Build history of the part. All positions in model axes, mm. Face numbers are marked on the shaded views. A direction names the side the tool comes from. Round coordinates to 2 decimals unless told otherwise and drop trailing zeros. Order: outer loops, then holes, each group sorted by start corner. A loop starts at its lowest first (then second) coordinate and runs counter-clockwise, first axis right, second up. Notation, with made-up numbers: (0, 56) -> (11, 56) arc R11 cw to (11, 69) -> close; hole circle Ø8 at (-36, 67). An arc over 180 degrees is marked (long way). Use a Markdown table: item, result. Add a question column.
Item 1: Probe L1, parallel to Y at x = 0, z = -2; L2, parallel to X at y = 7.5, z = 0.5; L3, parallel to Z at x = 15.5, y = 21.5. List the from-to ranges inside material, lowest first.
Item 2: Pin check, flat tips, straight feed: pin 1 (3 mm diameter, centred on x = -11, z = -2, fed in from +Y); pin 2 (2 mm diameter, centred on x = 9, z = 0.5, fed in from -Y); pin 3 (1 mm diameter, centred on x = 18, z = -0.5, fed in from -Y). Stop position of each tip, or through.
Item 3: Slice it at B-B, the plane x = 0. Give the cut face in (y, z), plus the area to 3 significant figures.
Item 4: Two-plate mould, pull along Y, no slides. Class the marked faces 1, 2 and 3: released by +Y, released by -Y, zero draft, split by the parting line, or undercut.
Item 5: Slice it at C-C, the plane y = 7. Give the cut face in (x, z).
Item 6: Slice it at A-A, the plane y = 0. Give the cut face in (x, z), plus the area to 3 significant figures.
Item 7: Slice it at D-D, the plane z = 2.25. Give the cut face in (x, y).
Item 8: 3-axis set-ups, long thin cutter, end or side, ignore diameter. For the marked faces 4 and 5: which of +Z, -Z, +X, -X, +Y, -Y reach the whole face in a straight line?
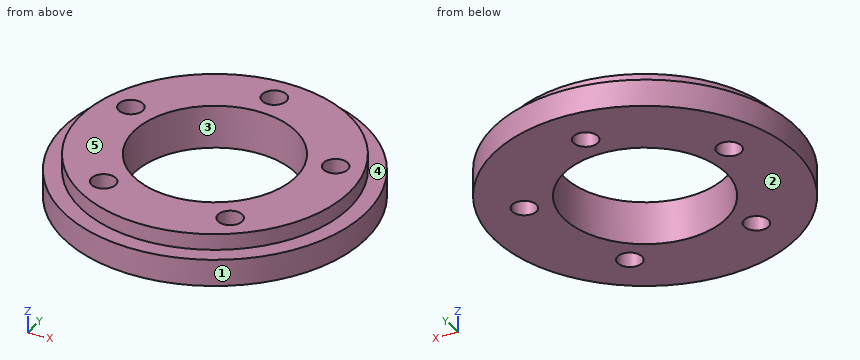
Autodesk Inventor part; units mm, degrees
ref_plane "YZ Plane" through (0, 0, 0) normal (1, 0, 0) x (0, 1, 0)
ref_plane "XZ Plane" through (0, 0, 0) normal (0, 1, 0) x (-1, 0, 0)
ref_plane "XY Plane" through (0, 0, 0) normal (0, 0, 1) x (1, 0, 0)
sketch "스케치1" plane through (0, 0, 0) normal (0, 0, 1) x (1, 0, 0)
  circle A0 centre (0, 0) radius 24.9
  circle A1 centre (0, 0) radius 28
  circle A2 centre (0, 0) radius 15
  dimension "d0" = 49.8
  dimension "d1" = 56
  dimension "d2" = 30
extrude "돌출1" add sketch "스케치1" along normal blind 3 contours A0
extrude "돌출2" add sketch "스케치1" against normal blind 5 contours A0 | A1
sketch "스케치3" plane through (0, 0, 3) normal (0, 0, 1) x (1, 0, 0)
  circle A0 centre (0, 0) radius 20 construction
  circle A1 centre (0, 20) radius 2.25
  circle A2 centre (-19.0211, 6.1803) radius 2.25
  circle A3 centre (-11.7557, -16.1803) radius 2.25
  circle A4 centre (11.7557, -16.1803) radius 2.25
  circle A5 centre (19.0211, 6.1803) radius 2.25
  dimension "d9" = 40
  dimension "d10" = 4.5
  dimension "d13" = 360
extrude "돌출3" cut sketch "스케치3" against normal blind 44.5
properties part number "사이클로이드 기어 축 연결 하우징"
Check sheet entries:
| question | item | result |
|---|---|---|
| 1 | L1 | -28 to -15, 15 to 17.75, 22.25 to 28 |
| 1 | L2 | -23.74 to -20.84, -17.2 to -12.99, 12.99 to 17.2, 20.84 to 23.74 |
| 1 | L3 | -5 to 0 |
| 2 | pin 1 | y = 26.34 |
| 2 | pin 2 | y = -26.79 |
| 2 | pin 3 | y = -21.86 |
| 3 | outline | (-28, -5) -> (-15, -5) -> (-15, 3) -> (-24.9, 3) -> (-24.9, 0) -> (-28, 0) -> close; (15, -5) -> (17.75, -5) -> (17.75, 3) -> (15, 3) -> close; (22.25, -5) -> (28, -5) -> (28, 0) -> (24.9, 0) -> (24.9, 3) -> (22.25, 3) -> close |
| 3 | area | 153 mm2 |
| 4 | face 1 | split by the parting line |
| 4 | face 2 | zero draft |
| 4 | face 3 | undercut |
| 5 | outline | (-27.11, -5) -> (-21.12, -5) -> (-21.12, 3) -> (-23.9, 3) -> (-23.9, 0) -> (-27.11, 0) -> close; (-16.93, -5) -> (-13.27, -5) -> (-13.27, 3) -> (-16.93, 3) -> close; (13.27, -5) -> (16.93, -5) -> (16.93, 3) -> (13.27, 3) -> close; (21.12, -5) -> (27.11, -5) -> (27.11, 0) -> (23.9, 0) -> (23.9, 3) -> (21.12, 3) -> close |
| 6 | outline | (-28, -5) -> (-15, -5) -> (-15, 3) -> (-24.9, 3) -> (-24.9, 0) -> (-28, 0) -> close; (15, -5) -> (28, -5) -> (28, 0) -> (24.9, 0) -> (24.9, 3) -> (15, 3) -> close |
| 6 | area | 189 mm2 |
| 7 | outline | circle Ø49.8 at (0, 0); hole circle Ø4.5 at (-19.02, 6.18); hole circle Ø30 at (0, 0); hole circle Ø4.5 at (-11.76, -16.18); hole circle Ø4.5 at (0, 20); hole circle Ø4.5 at (11.76, -16.18); hole circle Ø4.5 at (19.02, 6.18) |
| 8 | face 4 | +Z |
| 8 | face 5 | +Z, +X, -X, +Y, -Y |
